Could you check a few things on this drawing? It's one solid part, dimensions in mm from its lowest x, y, z. A direction names the side the tool comes from. Give positions to 0.01 mm unless a question says otherwise; leave off trailing zeros. Loops run counter-clockwise (first coordinate to the right, second up) from the corner with the lowest first, then second, coordinate; pieces in that order, holes last. Notation, with made-up numbers: (88.5, 37.5) -> (98.5, 37.5) arc R12 ccw to (98.5, 51.5) -> close; hole circle Ø11 at (82.5, 46.5). An arc over 180 degrees is marked (long way). Use CSV: the item, a comma, the result in double quotes.
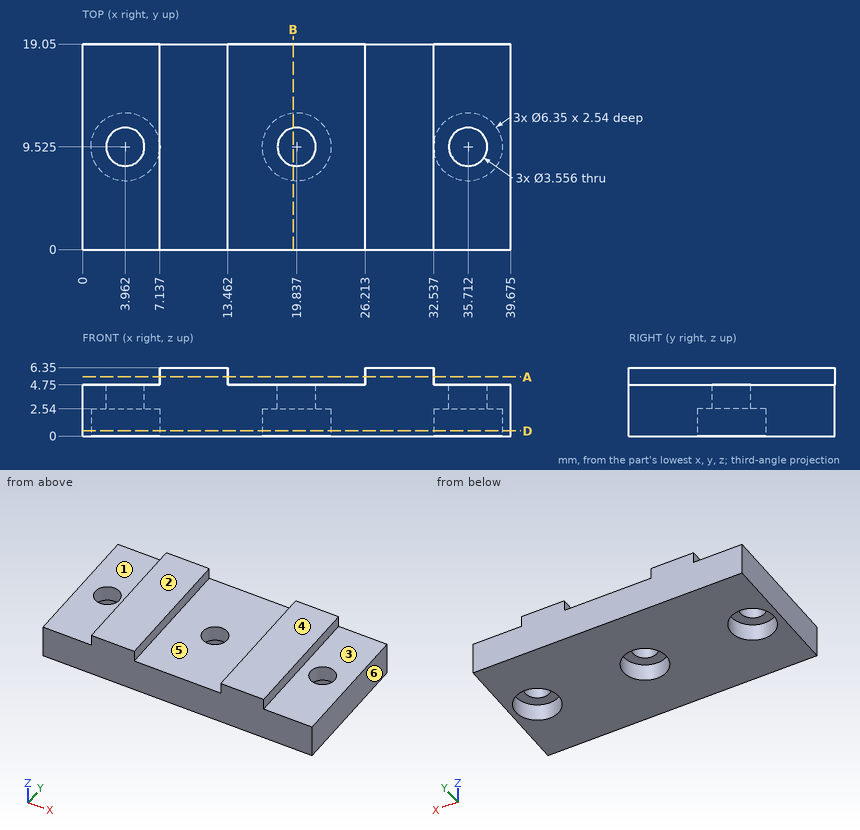
(1) If I drill on L1, parallel to X at y = 11, z = 3.5 (1 decimal); L2, parallel to Z at x = 23.5, y = 8; L3, parallel to X at y = 16.5, z = 5.25, over which ranges is the centre line in solid material (lowest first)? Write a range as from..to.
Answer sheet:
L1,"x = 0..3, 5..18.8, 20.8..34.7, 36.7..39.7"
L2,"z = 0..4.75"
L3,"x = 7.14..13.46, 26.21..32.54"
(2) If we section it at B-B, the plane x = 19.5: Write out the boundary of the cut face in (y, z).
Answer sheet:
outline,"(0, 0) -> (6.37, 0) -> (6.37, 2.54) -> (7.78, 2.54) -> (7.78, 4.75) -> (0, 4.75) -> close; (11.27, 2.54) -> (12.68, 2.54) -> (12.68, 0) -> (19.05, 0) -> (19.05, 4.75) -> (11.27, 4.75) -> close"
(3) If we section it at D-D, the plane z = 0.5: Give the number of separate pieces and of enclosed holes in the cut face, then the cut area to 3 significant figures.
Answer sheet:
separate pieces,"1"
enclosed holes,"3"
area,"661 mm2"
(4) If we section it at A-A, the plane z = 5.5: Write out the boundary of the cut face in (x, y), then the cut area to 3 significant figures.
Answer sheet:
outline,"(7.14, 0) -> (13.46, 0) -> (13.46, 19.05) -> (7.14, 19.05) -> close; (26.21, 0) -> (32.54, 0) -> (32.54, 19.05) -> (26.21, 19.05) -> close"
area,"241 mm2"
(5) Which directions (+Z, -Z, +X, -X, +Y, -Y) give clear straight access to the entire face, cutting with the end or side of a thin tool? Please do the marked faces 1, 2 and 3.
Answer sheet:
face 1,"+Z, -X, +Y, -Y"
face 2,"+Z, +X, -X, +Y, -Y"
face 3,"+Z, +X, +Y, -Y"
(6) Will these pins go through, and if not, where does the flat tip stop? pin 1 Ø5.5 at (x, y) = (35.71, 9.52) entering from +Z; pin 2 Ø3 at (x, y) = (19.84, 9.52) entering from +Z; pin 3 Ø1.3 at (y, z) = (5.5, 5.5) entering from +X; pin 4 Ø0.5 at (y, z) = (8, 5.5) entering from -X.
Answer sheet:
pin 1,"stops at z = 4.75"
pin 2,"passes through"
pin 3,"stops at x = 32.54"
pin 4,"stops at x = 7.14"
(7) We'd pull the mould along X, two halves only. Please class the marked faces 4, 5 and 6: released by +X, released by -X, zero draft, split by the parting line, or undercut.
Answer sheet:
face 4,"zero draft"
face 5,"undercut"
face 6,"released by +X"
